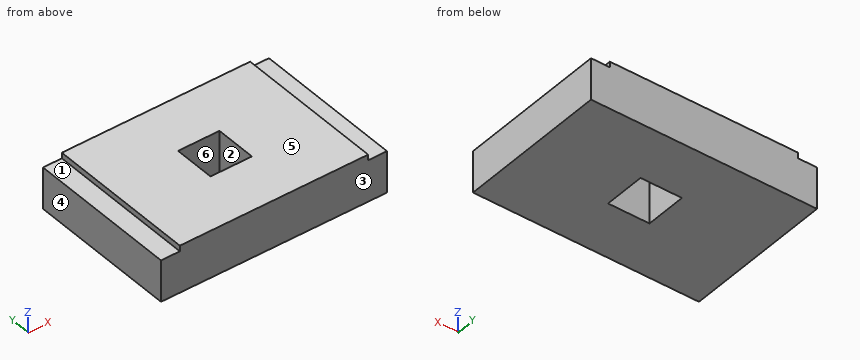
Solid Edge part; units mm, degrees
sketch "Sketch1" plane through (0, 0, 0) normal (0, -1, 0) x (1, 0, 0)
  line L0 (-60, 0) -> (-60, 22)
  line L1 (-60, 22) -> (-50, 22)
  line L2 (-50, 22) -> (-50, 25)
  line L3 (-50, 25) -> (50, 25)
  line L4 (50, 25) -> (50, 22)
  line L5 (50, 22) -> (60, 22)
  line L6 (60, 22) -> (60, 0)
  line L7 (60, 0) -> (-60, 0)
extrude "Protrusion1" add sketch "Sketch1" against normal blind 80
sketch "Sketch2" plane through (0, 40, 25) normal (0, 0, 1) x (1, 0, 0)
  line L0 (-11, -11) -> (11, -11)
  line L1 (11, -11) -> (11, 11)
  line L2 (11, 11) -> (-11, 11)
  line L3 (-11, 11) -> (-11, -11)
extrude "ExtrudedCutout_1" cut sketch "Sketch2" against normal blind 41.8556
Could you check a few things on this model? Use its own coordinates, in mm. Face numbers are marked on the shaded views. A direction names the side the tool comes from. Coordinates: 2 decimals unless noted, no trailing zeros. Order: outer loops, then holes, each group sorted by start corner. A loop starts at its lowest first (then second) coordinate and runs counter-clockwise, first axis right, second up. Notation, with made-up numbers: M 70,63.25 L 98,63.25 A21 cw 98,82.25 Z; hole C 18,-10 d7. An arc over 180 degrees is marked long. Use one line per item in the form item = value. Start each with the question number.
1. Suppose I cut it at A-A on x = 2. Write out the boundary of the cut face in (y, z).
2. Suppose I cut it at D-D on y = 53.5. Write out the boundary of the cut face in (x, z).
3. Suppose I cut it at B-B on y = 43. Write out the boundary of the cut face in (x, z).
4. We'd pull the mould along X, two halves only. Please class the marked faces 4, 5 and 6: +X half, -X half, draft (parallel to the pull), parting line (faces both ways), or undercut.
5. Please list where these lines run through material, in increasing order: line 1 (Y direction, x = 8.5, z = 9); line 2 (X direction, y = 49, z = 7.75); line 3 (X direction, y = 36, z = 23.25).
6. On a 3-axis mill with a long thin cutter (end or side, diameter ignored), from which of +Z, -Z, +X, -X, +Y, -Y can I reach the whole of each face in a straight line? I mean the marked faces 1, 2 and 3. Say none if no direction works.
7. Suppose I cut it at C-C on z = 8.5. Write out the boundary of the cut face in (x, y).
8. For pin 1 (3 mm diameter, centred on x = 53, y = 21, fed in from +Z); pin 2 (0.9 mm diameter, centred on y = 41.5, z = 23.5, fed in from -X); pin 3 (1.5 mm diameter, centred on y = 52.5, z = 23, fed in from +X), each with a flat end and sliding along its axis, tell me the tip position at first contact or that it passes through.
Geometry says:
q1.outline = M 0,0 L 29,0 L 29,25 L 0,25 Z; M 51,0 L 80,0 L 80,25 L 51,25 Z
q2.outline = M -60,0 L 60,0 L 60,22 L 50,22 L 50,25 L -50,25 L -50,22 L -60,22 Z
q3.outline = M -60,0 L -11,0 L -11,25 L -50,25 L -50,22 L -60,22 Z; M 11,0 L 60,0 L 60,22 L 50,22 L 50,25 L 11,25 Z
q4.face_4 = -X half
q4.face_5 = draft
q4.face_6 = undercut
q5.line_1 = 0 to 29, 51 to 80
q5.line_2 = -60 to -11, 11 to 60
q5.line_3 = -50 to -11, 11 to 50
q6.face_1 = +Z, -X, +Y, -Y
q6.face_2 = +Z, -Z
q6.face_3 = +Z, -Z, +X, -X, -Y
q7.outline = M -60,0 L 60,0 L 60,80 L -60,80 Z; hole M -11,29 L 11,29 L 11,51 L -11,51 Z
q8.pin_1 = 22
q8.pin_2 = -50
q8.pin_3 = 50
